Part model, mm, in its own coordinate system. A direction names the side the tool comes from. Give positions to 0.01 mm unless a question says otherwise; leave off trailing zeros. Order: outer loops, then holes, each group sorted by start corner. A loop starts at its lowest first (then second) coordinate and runs counter-clockwise, first axis right, second up. Notation, with made-up numbers: (6.5, -24.5) - (20.5, -24.5) arc R20 ccw to (20.5, 13.5) - close; hole circle Ø2 at (-23, 69.5). An arc over 180 degrees is marked (long way). One line per item, written item: value.
```python
from build123d import *

# Parameters (mm, degrees)
SALIENTE_EXTRUIR1_DEPTH = 4
REDONDEO1_R             = 0.5
REDONDEO2_R             = 1


with BuildPart() as part:
    # Croquis1 → Saliente-Extruir1 (new body)
    with BuildSketch(Plane(origin=(0, 0, 0), x_dir=(1, 0, 0), z_dir=(0, 1, 0))):
        Polygon((8.5, 2.5), (7, 2.5), (7, 12), (2.5, 12), (2.5, 16.5), (0, 16.5), (0, 0), (2.5, 0), (2.5, 4.5), (5, 4.5), (5, 0), (11, 0), (11, 16.5), (8.5, 16.5), align=None)
    extrude(amount=SALIENTE_EXTRUIR1_DEPTH)

    # Redondeo1
    redondeo1_edges = [part.edges().sort_by_distance(p)[0] for p in [
        (8.5, 2, -2.5),
        (0, 2, 0),
        (0, 2, -16.5),
        (7, 2, -12),
        (7, 2, -2.5),
    ]]
    fillet(redondeo1_edges, radius=REDONDEO1_R)

    # Redondeo2
    redondeo2_edges = [part.edges().sort_by_distance(p)[0] for p in [
        (11, 2, -16.5),
        (11, 2, 0),
    ]]
    fillet(redondeo2_edges, radius=REDONDEO2_R)


solid = part.part
```
1) Cut at A-A, the plane z = -2. Give the cut face in (x, y), then the cut area to 3 significant figures.
Outcome:
outline: (0, 0) - (2.5, 0) - (2.5, 4) - (0, 4) - close; (5, 0) - (11, 0) - (11, 4) - (5, 4) - close
area: 34.0 mm^2
2) Cut at C-C, the plane z = -6.75. Give the cut face in (x, y).
Outcome:
outline: (0, 0) - (7, 0) - (7, 4) - (0, 4) - close; (8.5, 0) - (11, 0) - (11, 4) - (8.5, 4) - close
3) Cut at D-D, the plane x = 4.75. Give the cut face in (y, z).
Outcome:
outline: (0, -12) - (4, -12) - (4, -4.5) - (0, -4.5) - close
4) Cut at B-B, the plane y = 2.4. Give the cut face in (x, z), then the cut area to 3 significant figures.
Outcome:
outline: (0, -16) arc R0.5 ccw to (0.5, -16.5) - (2.5, -16.5) - (2.5, -12) - (6.5, -12) arc R0.5 ccw to (7, -11.5) - (7, -3) arc R0.5 cw to (7.5, -2.5) - (8, -2.5) arc R0.5 cw to (8.5, -3) - (8.5, -16.5) - (10, -16.5) arc R1 ccw to (11, -15.5) - (11, -1) arc R1 ccw to (10, 0) - (5, 0) - (5, -4.5) - (2.5, -4.5) - (2.5, 0) - (0.5, 0) arc R0.5 ccw to (0, -0.5) - close
area: 129 mm^2
5) Mould opens along X. For faces 4 (the flat face through (5, 4, -8)), 5 (the flat face through (4, 2, -4.5)), 6 (the flat face through (0, 2, -8)) say: released by +X, released by -X, zero draft, split by the parting line, or undercut.
Outcome:
face 4: zero draft
face 5: undercut
face 6: released by -X
6) Which spindle directions (+Z, -Z, +X, -X, +Y, -Y) get a long thin tool onto all of the face, cutting with end or side? Do faces 1 (the flat face through (7, 2, 0)), 2 (the flat face through (7, 2, -7)), 3 (the flat face through (5, 2, -2)). Say none if no direction does.
Outcome:
face 1: +Z, +X, -X, +Y, -Y
face 2: -Z, +Y, -Y
face 3: +Z, +Y, -Y
7) Pin check, flat tips, straight feed: pin 1 (0.8 mm diameter, centred on x = 4, y = 1.5, fed in from +Z); pin 2 (5 mm diameter, centred on x = 5.5, z = -10.5, fed in from -Y); pin 3 (2 mm diameter, centred on x = 4.5, y = 1.5, fed in from -Z). Stop position of each tip, or through.
Outcome:
pin 1: stops at z = -4.5
pin 2: stops at y = 0
pin 3: stops at z = -12
8) Drill centre lines: line 1 along X through (y, z) = (3.1, -3.5); line 2 along X through (y, z) = (3.45, -2.25); line 3 along X through (y, z) = (0.5, -12.5). Where is each one in solid material? Low to high. Write a range as from..to.
Outcome:
line 1: x = 0..2.5, 5..7, 8.5..11
line 2: x = 0..2.5, 5..11
line 3: x = 0..2.5, 8.5..11
